from build123d import *

# Parameters (mm, degrees)
CROQUIS1_R              = 9.875
CROQUIS1_W              = 5
CROQUIS1_H              = 5
SALIENTE_EXTRUIR1_DEPTH = 3
REDONDEO1_R             = 1
CROQUIS2_R              = 10.5
CORTAR_EXTRUIR1_DEPTH   = 10


with BuildPart() as part:
    # Croquis1 → Saliente-Extruir1 (new body)
    with BuildSketch(Plane.XY):
        Circle(CROQUIS1_R)
        with BuildLine():
            ThreePointArc((9.875, 0), (0, -9.875), (-9.875, 0))
            Line((-9.875, 0), (-9.875, -10.4))
            Line((-9.875, -10.4), (-9.875, -15.4))
            Line((-9.875, -15.4), (-9.875, -25.4))
            Line((-9.875, -25.4), (9.875, -25.4))
            Line((9.875, -25.4), (9.875, -15.4))
            Line((9.875, -15.4), (9.875, -10.4))
            Line((9.875, -10.4), (9.875, 0))
        make_face()
        with Locations((12.375, -12.9)):
            Rectangle(CROQUIS1_W, CROQUIS1_H)
        with Locations((-12.375, -12.9)):
            Rectangle(CROQUIS1_W, CROQUIS1_H)
    extrude(amount=SALIENTE_EXTRUIR1_DEPTH)

    # Redondeo1
    redondeo1_edges = [part.edges().sort_by_distance(p)[0] for p in [
        (0, -25.4, 3),
    ]]
    fillet(redondeo1_edges, radius=REDONDEO1_R)

    # Croquis2 → Cortar-Extruir1 (cut)
    with BuildSketch(Plane.XY.offset(3)):
        Circle(CROQUIS2_R)
    extrude(amount=-CORTAR_EXTRUIR1_DEPTH, mode=Mode.SUBTRACT)


solid = part.part
Geometry: final body of the model. Coordinates: model frame, mm. A direction names the side the tool comes from. Coordinates: 2 decimals unless noted, no trailing zeros. Order: outer loops, then holes, each group sorted by start corner. A loop starts at its lowest first (then second) coordinate and runs counter-clockwise, first axis right, second up.
(1) Section query A-A (z = 0.7). Return the cut outline in (x, y) (3 decimals).
(2) Draft query along X for faces 4 (the face through (9.875, -20, 1)), 5 (the face through (-14.875, -13, 1)), 6 (the face through (-0.2, -10.5, 1.5)), 7 (the face through (0, -25.4, 1)). Return one class per face: pulls with the +X half, pulls with the -X half, needs draft (parallel to the pull), parting line crosses it, or undercut.
(3) Section query C-C (x = -2). Return the cut outline in (y, z).
(4) Section query D-D (y = -22.75). Return the cut outline in (x, z) (3 decimals).
(5) Access query for faces 1 (the face through (-12, -10.4, 1)), 2 (the face through (12, -10.4, 1)), 3 (the face through (-9.875, -20, 1)). Directions: +Z, -Z, +X, -X, +Y, -Y. A direction counts if a zero-diameter tool reaches every point of the face in a straight line with its end or side. Return the directions, or none.
(6) Material intervals for probe 1 along Y at (x, z) = (10, 1.6); probe 2 along X at (y, z) = (-18.5, 2.6) (3 decimals); probe 3 along X at (y, z) = (-6, 0.6) (3 decimals), sorted ascending.
(7) First-contact query: pin 1 (1.5 mm diameter, centred on x = 13, z = 1.5, fed in from +Y); pin 2 (1.5 mm diameter, centred on y = -15.5, z = 1, fed in from +X) (3 decimals). Flat tips, straight axial feed; report the tip coordinate or a pass-through.
(8) Section query B-B (y = -8.5). Return the cut outline in (x, z) (3 decimals), plus the area to 3 significant figures.
Solution:
1. outline: (-14.875, -15.4) - (-9.875, -15.4) - (-9.875, -25.4) - (9.875, -25.4) - (9.875, -15.4) - (14.875, -15.4) - (14.875, -10.4) - (9.875, -10.4) - (9.875, -3.569) arc R10.5 cw to (-9.875, -3.569) - (-9.875, -10.4) - (-14.875, -10.4) - close
2. face 4: pulls with the +X half
2. face 5: pulls with the -X half
2. face 6: undercut
2. face 7: needs draft
3. outline: (-25.4, 0) - (-10.31, 0) - (-10.31, 3) - (-24.4, 3) arc R1 ccw to (-25.4, 2) - close
4. outline: (-9.875, 0) - (9.875, 0) - (9.875, 3) - (-9.875, 3) - close
5. face 1: +Z, -Z, -X, +Y
5. face 2: +Z, -Z, +X, +Y
5. face 3: +Z, -Z, -X, -Y
6. probe 1: y = -15.4 to -10.4
6. probe 2: x = -9.875 to 9.875
6. probe 3: x = -9.875 to -8.617, 8.617 to 9.875
7. pin 1: stops at y = -10.4
7. pin 2: stops at x = 14.875
8. outline: (-9.875, 0) - (-6.164, 0) - (-6.164, 3) - (-9.875, 3) - close; (6.164, 0) - (9.875, 0) - (9.875, 3) - (6.164, 3) - close
8. area: 22.3 mm2
